from build123d import *

# Parameters (mm, degrees)
SKETCH1_W           = 48
SKETCH1_H           = 48
BOSS_EXTRUDE1_DEPTH = 33
SHELL1_T            = -4
SKETCH2_W           = 40
SKETCH2_H           = 8
CUT_EXTRUDE1_DEPTH  = 49
SKETCH3_R           = 2
BOSS_EXTRUDE2_DEPTH = 5


with BuildPart() as part:
    # Sketch1 → Boss-Extrude1 (new body)
    with BuildSketch(Plane.XY):
        Rectangle(SKETCH1_W, SKETCH1_H)
    extrude(amount=BOSS_EXTRUDE1_DEPTH)

    # Shell1
    shell1_openings = [part.faces().sort_by_distance(p)[0] for p in [
        (0, 0, 33),
    ]]
    offset(amount=SHELL1_T, openings=shell1_openings, kind=Kind.INTERSECTION)

    # Sketch2 → Cut-Extrude1 (cut, through all)
    with BuildSketch(Plane(origin=(0, 24, 0), x_dir=(1, 0, 0), z_dir=(0, 1, 0))):
        with Locations((0, -8)):
            Rectangle(SKETCH2_W, SKETCH2_H)
    extrude(amount=-CUT_EXTRUDE1_DEPTH, mode=Mode.SUBTRACT)

    # Sketch3 → Boss-Extrude2 (add)
    with BuildSketch(Plane(origin=(24, 0, 0), x_dir=(0, 0, -1), z_dir=(1, 0, 0))):
        with Locations((-10, 0)):
            Circle(SKETCH3_R)
    boss_extrude2 = extrude(amount=BOSS_EXTRUDE2_DEPTH)

    # Mirror1: Boss-Extrude2 across plane
    add(boss_extrude2.mirror(Plane(origin=(0, 0, 0), x_dir=(0, 0, 1), z_dir=(1, 0, 0))))


solid = part.part
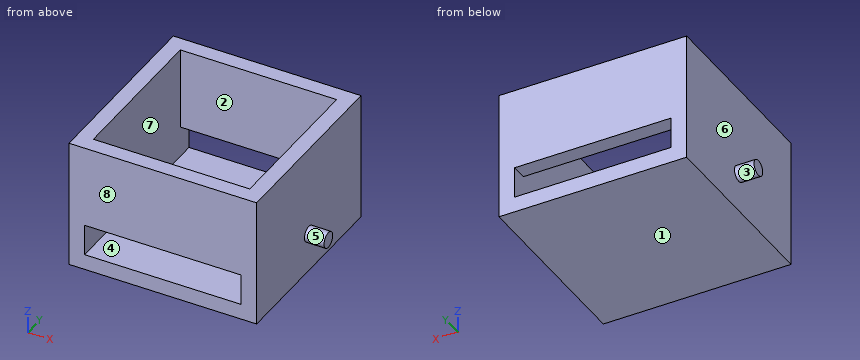
Could you check a few things on this model? Use its own coordinates, in mm. Face numbers are marked on the shaded views. A direction names the side the tool comes from. Coordinates: 2 decimals unless noted, no trailing zeros. Order: outer loops, then holes, each group sorted by start corner. A loop starts at its lowest first (then second) coordinate and runs counter-clockwise, first axis right, second up.
Q1. Thinking about a two-plate mould opening in Y: for the marked faces 6, 7 and 8, which applies, released by +Y, released by -Y, zero draft, split by the parting line, or undercut?
Q2. Please list where these lines run through material, in increasing order: L1, parallel to X at y = 6, z = 9.5; L2, parallel to Z at x = 3, y = 21.5.
Q3. Suppose I cut it at C-C on z = 25.5. Please give me the cut outline in (x, y), and give its area (3 significant figures).
Q4. Suppose I cut it at A-A on x = 5. Please give me the cut outline in (y, z), and give its area (3 significant figures).
Q5. Suppose I cut it at B-B on z = 6.5. Please give me the cut outline in (x, y), and give its area (3 significant figures).
Q6. Which directions (+Z, -Z, +X, -X, +Y, -Y) give clear straight access to the entire face, cutting with the end or side of a thin tool? Please do the marked faces 1, 2, 3, 4 and 5.
Q7. Will these pins go through, and if not, where does the flat tip stop? pin 1 (2 mm diameter, centred on x = -2.5, y = -19, fed in from -Z); pin 2 (12 mm diameter, centred on x = 10, y = -6, fed in from +Z); pin 3 (12 mm diameter, centred on y = 8, z = 13, fed in from +X); pin 4 (14.5 mm diameter, centred on y = 10, z = 24.5, fed in from -X).
Q8. Suppose I cut it at D-D on y = 0. Please give me the cut outline in (x, z), and give its area (3 significant figures).
Answer:
1. face 6: zero draft
1. face 7: undercut
1. face 8: released by -Y
2. L1: x = -24 to -20, 20 to 24
2. L2: z = 0 to 4, 12 to 33
3. outline: (-24, -24) - (24, -24) - (24, 24) - (-24, 24) - close; hole (-20, -20) - (20, -20) - (20, 20) - (-20, 20) - close
3. area: 704 mm2
4. outline: (-24, 0) - (24, 0) - (24, 4) - (-24, 4) - close; (-24, 12) - (-20, 12) - (-20, 33) - (-24, 33) - close; (20, 12) - (24, 12) - (24, 33) - (20, 33) - close
4. area: 360 mm2
5. outline: (-24, -24) - (-20, -24) - (-20, 24) - (-24, 24) - close; (20, -24) - (24, -24) - (24, 24) - (20, 24) - close
5. area: 384 mm2
6. face 1: -Z, +X, -X, +Y, -Y
6. face 2: +Z
6. face 3: -X
6. face 4: +Y, -Y
6. face 5: +X
7. pin 1: stops at z = 0
7. pin 2: stops at z = 4
7. pin 3: stops at x = 24
7. pin 4: stops at x = -24
8. outline: (-29, 8) - (-24, 8) - (-24, 0) - (24, 0) - (24, 8) - (29, 8) - (29, 12) - (24, 12) - (24, 33) - (20, 33) - (20, 4) - (-20, 4) - (-20, 33) - (-24, 33) - (-24, 12) - (-29, 12) - close
8. area: 464 mm2
